from build123d import *

# Parameters (mm, degrees)
EXTRUDE_1_DEPTH     = 0.6
EXTRUDE_START       = 9
EXTRUDE_3_DEPTH     = 9
EXTRUDE_START_2     = 0.6
EXTRUDE_4_DEPTH     = 0.6
FILLET_1_R          = 1
FILLET_2_R          = 1
CUT_EXTRUDE_1_DEPTH = 1.5


with BuildPart() as part:
    # Sketch 1 → Extrude 1 (new body)
    with BuildSketch(Plane(origin=(0, 0, 0), x_dir=(1, 0, 0), z_dir=(0, 1, 0))):
        with BuildLine():
            Line((13.895707880639236, -1.0302631578947374), (10.575971038533972, -9.071988551065596))
            Line((10.575971038533972, -9.071988551065596), (6.899999999999973, -11.951150572225266))
            ThreePointArc((6.899999999999973, -11.951150572225266), (-12.749537548655752, 5.281031366638245), (13.329776402789136, 3.571702822414798))
            Line((13.329776402789136, 3.571702822414798), (13.895707880639236, -1.0302631578947374))
        make_face()
        with BuildLine():
            Line((11.4, 7e-16), (8.080263157894738, -8.041725393170857))
            ThreePointArc((8.080263157894738, -8.041725393170857), (-10.53743327381009, 4.3500000000000005), (11.4, 7e-16))
        make_face(mode=Mode.SUBTRACT)
    extrude(amount=EXTRUDE_1_DEPTH)

    # Sketch 2 → Extrude 3 (add)
    with BuildSketch(Plane(origin=(0, 0, 0), x_dir=(-1, 0, 0), z_dir=(0, -1, 0)).offset(EXTRUDE_START)):
        with BuildLine():
            Line((-13.895707880639238, -1.0302631578947372), (-10.575971038533975, -9.071988551065594))
            Line((-10.575971038533975, -9.071988551065594), (-6.90000000000001, -11.951150572225243))
            ThreePointArc((-6.90000000000001, -11.951150572225243), (12.749537548655738, 5.281031366638277), (-13.329776402789168, 3.5717028224146974))
            Line((-13.329776402789168, 3.5717028224146974), (-13.895707880639238, -1.0302631578947372))
        make_face()
        with BuildLine():
            Line((-9.448115747583758, -8.635572292573311), (-12.787098442057127, -0.5745549870466524))
            ThreePointArc((-12.787098442057127, -0.5745549870466524), (11.825658016144468, 4.89834793427316), (-9.448115747583758, -8.635572292573311))
        make_face(mode=Mode.SUBTRACT)
    extrude(amount=-EXTRUDE_3_DEPTH)

    # Sketch 5 → Extrude 4 (add)
    # profile 1 of 2: a face of its own
    with BuildSketch(Plane(origin=(0, -9, 0), x_dir=(-1, 0, 0), z_dir=(0, -1, 0)).offset(EXTRUDE_START_2)):
        with BuildLine():
            Line((-10.575971038533975, -9.071988551065594), (-6.90000000000001, -11.951150572225243))
            ThreePointArc((-6.90000000000001, -11.951150572225243), (12.749537548655738, 5.281031366638277), (-13.329776402789168, 3.5717028224146974))
            Line((-13.329776402789168, 3.5717028224146974), (-13.895707880639238, -1.0302631578947372))
            Line((-13.895707880639238, -1.0302631578947372), (-10.575971038533975, -9.071988551065594))
        make_face()
        with BuildLine():
            ThreePointArc((-12.787098442057129, -0.5745549870466533), (11.825658016144468, 4.898347934273158), (-9.448115747583758, -8.635572292573311))
            Line((-9.448115747583758, -8.635572292573311), (-12.787098442057129, -0.5745549870466533))
        make_face(mode=Mode.SUBTRACT)
    # profile 2 of 2: a face of its own
    with BuildSketch(Plane(origin=(0, -9, 0), x_dir=(-1, 0, 0), z_dir=(0, -1, 0)).offset(EXTRUDE_START_2)):
        with BuildLine():
            Line((-9.448115747583758, -8.635572292573311), (-12.787098442057129, -0.5745549870466533))
            ThreePointArc((-12.787098442057129, -0.5745549870466533), (11.825658016144468, 4.898347934273158), (-9.448115747583758, -8.635572292573311))
        make_face()
        with BuildLine():
            ThreePointArc((-8.08026315789474, -8.041725393170857), (10.537433273810091, 4.35), (-11.400000000000002, 8.7e-16))
            Line((-11.400000000000002, 8.7e-16), (-8.08026315789474, -8.041725393170857))
        make_face(mode=Mode.SUBTRACT)
    extrude(amount=-EXTRUDE_4_DEPTH)

    # Fillet 1
    # the kernel refuses this fillet: 1 mm, written as the material it takes off along each edge
    with BuildSketch(Plane(origin=(12.54413178302016, -9.6, 7.530449293095305), x_dir=(2.4e-16, 1, 3.1e-16), z_dir=(-0.7872642977944737, 0, 0.6166157031881158))) as fillet_1_piece_1:
        with BuildLine():
            CenterArc((FILLET_1_R, FILLET_1_R), FILLET_1_R, 180, 90)
            Line((-4e-16, FILLET_1_R), (0, 0))
            Line((0, 0), (FILLET_1_R, 0))
        make_face()
    extrude(amount=9.669297272634138, mode=Mode.SUBTRACT)
    with BuildSketch(Plane(origin=(3.55e-15, -9.6, -4.88e-15), x_dir=(0.6484067938631516, 0, 0.7612940494133056), z_dir=(0.7612940494133056, 0, -0.6484067938631516))) as fillet_1_piece_2:
        with BuildLine():
            CenterArc((13.8 - FILLET_1_R, -FILLET_1_R), FILLET_1_R, 0, 90)
            Line((13.8 - FILLET_1_R, 0), (13.8, 0))
            Line((13.8, 0), (13.8, -FILLET_1_R))
        make_face()
    revolve(axis=Axis((3.55e-15, -9.6, -4.88e-15), (0, -1, 0)), revolution_arc=305.8431767721365, mode=Mode.SUBTRACT)
    with BuildSketch(Plane(origin=(13.024635027269708, -9.6, -6.05301069145193), x_dir=(-0.9925231476148944, 0, 0.12205655020777262), z_dir=(0.12205655020777263, 0, 0.9925231476148945))) as fillet_1_piece_3:
        with BuildLine():
            CenterArc((FILLET_1_R, -FILLET_1_R), FILLET_1_R, 90, 90)
            Line((1.65e-15, -FILLET_1_R), (0, 0))
            Line((0, 0), (FILLET_1_R, 0))
        make_face()
    extrude(amount=9.636633403833748, mode=Mode.SUBTRACT)
    with BuildSketch(Plane(origin=(14.849655249060289, -9.6, -1.2805774723267747), x_dir=(0, 1, 0), z_dir=(-0.381578947368421, 0, 0.9243362520886044))) as fillet_1_piece_4:
        with BuildLine():
            CenterArc((FILLET_1_R, FILLET_1_R), FILLET_1_R, 180, 90)
            Line((0, FILLET_1_R), (0, 0))
            Line((0, 0), (FILLET_1_R, 0))
        make_face()
    extrude(amount=13.700000000000005, mode=Mode.SUBTRACT)

    # Fillet 2
    # the kernel refuses this fillet: 1 mm, written as the material it takes off along each edge
    with BuildSketch(Plane(origin=(13.024635027269696, 0.6, -6.053010691452034), x_dir=(0, -1, 0), z_dir=(0.12205655020777641, 0, 0.992523147614894))) as fillet_2_piece_1:
        with BuildLine():
            CenterArc((FILLET_2_R, -FILLET_2_R), FILLET_2_R, 90, 89.99999999999991)
            Line((-1.1e-16, -FILLET_2_R), (0, 0))
            Line((0, 0), (FILLET_2_R, 0))
        make_face()
    extrude(amount=9.636633403833853, mode=Mode.SUBTRACT)
    with BuildSketch(Plane(origin=(1e-15, 0.6, -1.55e-15), x_dir=(0.6484067938631493, 0, 0.7612940494133076), z_dir=(0.7612940494133076, 0, -0.6484067938631493))) as fillet_2_piece_2:
        with BuildLine():
            CenterArc((13.799999999999997 - FILLET_2_R, FILLET_2_R), FILLET_2_R, 270, 90)
            Line((13.799999999999997 - FILLET_2_R, -1.1e-16), (13.799999999999997, 0))
            Line((13.799999999999997, 0), (13.799999999999997, FILLET_2_R))
        make_face()
    revolve(axis=Axis((1e-15, 0.6, -1.55e-15), (0, -1, 0)), revolution_arc=305.84317677213596, mode=Mode.SUBTRACT)
    with BuildSketch(Plane(origin=(12.544131783020157, 0.6, 7.530449293095308), x_dir=(-0.616615703188115, 0, -0.7872642977944742), z_dir=(-0.7872642977944742, 0, 0.616615703188115))) as fillet_2_piece_3:
        with BuildLine():
            CenterArc((FILLET_2_R, FILLET_2_R), FILLET_2_R, 180, 90)
            Line((0, FILLET_2_R), (0, 0))
            Line((0, 0), (FILLET_2_R, 0))
        make_face()
    extrude(amount=9.669297272634177, mode=Mode.SUBTRACT)
    with BuildSketch(Plane(origin=(14.849655249060289, 0.6, -1.2805774723267738), x_dir=(-0.9243362520886041, 0, -0.3815789473684211), z_dir=(-0.38157894736842113, 0, 0.9243362520886043))) as fillet_2_piece_4:
        with BuildLine():
            CenterArc((FILLET_2_R, FILLET_2_R), FILLET_2_R, 180, 90)
            Line((1.7e-16, FILLET_2_R), (0, 0))
            Line((0, 0), (FILLET_2_R, 0))
        make_face()
    extrude(amount=13.700000000000005, mode=Mode.SUBTRACT)

    # Sketch 7 → Cut-Extrude 1 (cut)
    with BuildSketch(Plane(origin=(9.740131578947372, 0, 4.0208626965854295), x_dir=(-0.381578947368421, 0, 0.9243362520886043), z_dir=(-0.9243362520886043, 0, -0.381578947368421))):
        Polygon((-4.350000000000001, 0.6), (-4.350000000000001, 0), (4.349999999999998, 2.66e-15), (4.349999999999998, 0.6000000000000028), align=None)
    extrude(amount=-CUT_EXTRUDE_1_DEPTH, mode=Mode.SUBTRACT)


solid = part.part
Build history of the part. All positions in model axes, mm. A direction names the side the tool comes from. Coordinates: 2 decimals unless noted, no trailing zeros. Order: outer loops, then holes, each group sorted by start corner. A loop starts at its lowest first (then second) coordinate and runs counter-clockwise, first axis right, second up. Notation, with made-up numbers: (-3, -34) - (8, -34) arc R27 cw to (8, -5) - close; hole circle Ø7 at (-33, -40). An arc over 180 degrees is marked (long way). Put each result on its own line as item: value.
1. Saw through at A-A (x = 0). Write the cut outline in (y, z).
Answer sheet:
outline: (-9.6, -12.8) arc R1 ccw to (-8.6, -13.8) - (-0.4, -13.8) arc R1 ccw to (0.6, -12.8) - (0.6, -11.4) - (0, -11.4) - (0, -12.8) - (-9, -12.8) - (-9, -11.4) - (-9.6, -11.4) - close; (-9.6, 11.4) - (-9, 11.4) - (-9, 12.8) - (0, 12.8) - (0, 11.4) - (0.6, 11.4) - (0.6, 12.8) arc R1 ccw to (-0.4, 13.8) - (-8.6, 13.8) arc R1 ccw to (-9.6, 12.8) - close
2. Drop flat-ended pins along their axis: P1, Ø1.4, axis at x = 11.5, z = 6.5, coming from the +Y side (3 decimals); P2, Ø3, axis at x = 8.5, y = -5.5, coming from the +Z side; P3, Ø6, axis at y = -1.5, z = 3.5, coming from the -X side; P4, Ø13.5, axis at x = 0, z = 0, coming from the -Y side. Give the stop position or say it passes through.
Answer sheet:
P1: stops at y = 0.585
P2: stops at z = 11.87
P3: stops at x = -13.79
P4: passes through
3. Tool access for faces 1 (the face through (-8, 0, -9)), 2 (the face through (13.31, -9.315, -1.266)), 3 (the face through (8.588, 0.299, 10.267)), 4 (the face through (11.15, 0.3, 4.54)), 5 (the face through (9.763, -9.304, 3.965)): list every direction of +Z, -Z, +X, -X, +Y, -Y with a clear straight run to the whole face (end or side of a thin tool).
Answer sheet:
face 1: none
face 2: -Z, +X, -Y
face 3: +Z, +X, +Y
face 4: +Y
face 5: +Y, -Y
4. Probe line 1 along Z through (x, y) = (0, -3.75); line 2 along Z through (x, y) = (-8.5, -3); line 3 along Y through (x, z) = (-2.75, -11.75). List the from-to ranges inside material, lowest first. Write a range as [from, to].
Answer sheet:
line 1: z = [-13.8, -12.8], [12.8, 13.8]
line 2: z = [-10.87, -9.57], [9.57, 10.87]
line 3: y = [-9.6, -9], [0, 0.6]
5. Pull direction Y, two halves, no side cores. Call faces 6 (the face through (10, -9.6, 5)), 7 (the face through (-9, -9, 8)), 8 (the face through (13.326, 0.299, -1.268)): pulls with the +Y half, pulls with the -Y half, needs draft (parallel to the pull), parting line crosses it, or undercut.
Answer sheet:
face 6: pulls with the -Y half
face 7: undercut
face 8: pulls with the +Y half
6. Saw through at B-B (y = -6). Write the cut outline in (x, z), and give its area (3 significant figures).
Answer sheet:
outline: (6.9, 11.95) arc R13.8 ccw (long way) to (13.33, -3.57) - (13.9, 1.03) - (10.58, 9.07) - close; hole (9.45, 8.64) arc R12.8 ccw (long way) to (12.79, 0.57) - close
area: 84.6 mm^2
